Autodesk Inventor part; units mm, degrees
ref_plane "Work Plane2" through (31.1532, -17.5901, -37) normal (0.7071, 0.7071, 0) x (-0.7071, 0.7071, 0)
ref_plane "Work Plane4" through (0.92, 19.6401, -37) normal (-1, 0, 0) x (0, 0, -1)
ref_plane "YZ Plane" through (0, 0, 0) normal (1, 0, 0) x (0, 1, 0)
sketch "Sketch1" plane through (0, 0, 0) normal (0, 0, 1) x (1, 0, 0)
  line L0 (0, 0) -> (0, 7.4776)
  line L1 (0, 7.4776) -> (-5.7, 7.4776)
  line L2 (-5.7, 7.4776) -> (-21.2563, -8.0788)
  line L3 (-21.2563, -8.0788) -> (-21.2563, -11.0788)
  line L4 (-21.2563, -11.0788) -> (-20.5492, -11.7859)
  line L5 (-20.5492, -11.7859) -> (-21.2563, -12.493)
  line L6 (-21.2563, -12.493) -> (-19.7664, -13.983)
  line L7 (-19.7664, -13.983) -> (-25.1404, -19.357)
  line L8 (-25.1404, -19.357) -> (-27.1017, -19.2987)
  line L9 (-27.1017, -19.2987) -> (-27.8088, -20.0059)
  line L10 (-27.8088, -20.0059) -> (-23.0005, -24.8142)
  line L11 (-23.0005, -24.8142) -> (-3.2015, -5.0152)
  line L12 (-1.88, 9.6426) -> (-1.2574, 11.8658)
  line L13 (-1.2574, 11.8658) -> (-2.8574, 11.8658)
  line L14 (-2.8574, 11.8658) -> (-5.5444, 9.1788)
  line L15 (-23.5149, -7.7918) -> (-6.5444, 9.1788)
  line L16 (-6.5444, 9.1788) -> (-5.5444, 9.1788)
  line L17 (-23.5149, -7.7918) -> (-23.5149, -11.7918)
  line L18 (-29.3132, -17.5901) -> (-23.5149, -11.7918)
  line L19 (-29.3132, -17.5901) -> (-30.4446, -16.4587)
  line L20 (-30.4446, -16.4587) -> (-29.4153, -15.4295)
  line L21 (-29.4153, -15.4295) -> (-30.1224, -14.7223)
  line L22 (-30.1224, -14.7223) -> (-32.668, -17.2679)
  line L23 (-32.668, -17.2679) -> (-22.9298, -27.0062)
  line L24 (-22.9298, -27.0062) -> (-1.4337, -5.5102)
  line L25 (0.92, 16.812) -> (0.92, -19.9546) construction
  line L26 (1.84, 0) -> (1.84, 7.4776)
  line L27 (1.84, 7.4776) -> (7.54, 7.4776)
  line L28 (7.54, 7.4776) -> (23.0963, -8.0788)
  line L29 (23.0963, -8.0788) -> (23.0963, -11.0788)
  line L30 (23.0963, -11.0788) -> (22.3892, -11.7859)
  line L31 (22.3892, -11.7859) -> (23.0963, -12.493)
  line L32 (23.0963, -12.493) -> (21.6064, -13.983)
  line L33 (21.6064, -13.983) -> (26.9804, -19.357)
  line L34 (26.9804, -19.357) -> (28.9417, -19.2987)
  line L35 (28.9417, -19.2987) -> (29.6488, -20.0059)
  line L36 (29.6488, -20.0059) -> (24.8405, -24.8142)
  line L37 (24.8405, -24.8142) -> (5.0415, -5.0152)
  line L38 (3.72, 9.6426) -> (3.0974, 11.8658)
  line L39 (3.0974, 11.8658) -> (4.6974, 11.8658)
  line L40 (4.6974, 11.8658) -> (7.3844, 9.1788)
  line L41 (25.3549, -7.7918) -> (8.3844, 9.1788)
  line L42 (8.3844, 9.1788) -> (7.3844, 9.1788)
  line L43 (25.3549, -7.7918) -> (25.3549, -11.7918)
  line L44 (31.1532, -17.5901) -> (25.3549, -11.7918)
  line L45 (31.1532, -17.5901) -> (32.2846, -16.4587)
  line L46 (32.2846, -16.4587) -> (31.2553, -15.4295)
  line L47 (31.2553, -15.4295) -> (31.9624, -14.7223)
  line L48 (31.9624, -14.7223) -> (34.508, -17.2679)
  line L49 (34.508, -17.2679) -> (24.7698, -27.0062)
  line L50 (24.7698, -27.0062) -> (3.2737, -5.5102)
  line L51 (-1.88, 9.6426) -> (3.72, 9.6426)
  arc A0 (3.2737, -5.5102) -> (-1.4337, -5.5102) centre (0.92, -4.1167) ccw
  arc A1 (5.0415, -5.0152) -> (1.84, 0) centre (0.92, -4.1167) ccw
  arc A2 (0, 0) -> (-3.2015, -5.0152) centre (0.92, -4.1167) ccw
  point P0 (-22.4534, -16.67)
  dimension "d1" = 5.7
  dimension "d2" = 135
  dimension "d3" = 22
  dimension "d13" = 3
  dimension "d14" = 28
  dimension "d22" = 1.6
  dimension "d23" = 3.8
  dimension "d24" = 1
  dimension "d25" = 24
  dimension "d30" = 4
  dimension "d34" = 3.6
  dimension "d36" = 1.5
  dimension "d38" = 1.6
  dimension "d47" = 1.84
  dimension "d55" = 8.2
  dimension "d56" = 1.6
  dimension "d57" = 1
  dimension "d59" = 7.6
  dimension "d61" = 1
  dimension "d62" = 6.8
  dimension "d72" = 30.4
  dimension "d74" = 13.772
  dimension "d75" = 4.2
  dimension "d76" = 5.6
  dimension "d77" = 1.8
  dimension "d78" = 1
  dimension "d80" = 90
  dimension "d89" = 7.4776
extrude "Extrusion1" add sketch "Sketch1" against normal blind 37
ref_plane "Work Plane2" through (31.1532, -17.5901, -37) normal (0.7071, 0.7071, 0) x (-0.7071, 0.7071, 0)
sketch "Sketch3" plane through (31.1532, -17.5901, -37) normal (0.7071, 0.7071, 0) x (-0.7071, 0.7071, 0)
  circle A0 centre (5.2, 18.5) radius 3
  line L0 (0, 37) -> (8.2, 37)
  line L1 (8.2, 37) -> (8.2, 0)
  point P0 (34.4667, 37)
  dimension "d65" = 18.5
  dimension "d67" = 6
extrude "Extrusion2" cut sketch "Sketch3" against normal blind 6
thread "Thread1"
ref_plane "Work Plane4" through (0.92, 19.6401, -37) normal (-1, 0, 0) x (0, 0, -1)
mirror "Mirror2" about plane through (0.92, 19.6401, -37) normal (-1, 0, 0) of "Extrusion2"
thread "Thread2"
sketch "Sketch4" plane through (31.1532, -17.5901, -37) normal (0.7071, 0.7071, 0) x (-0.7071, 0.7071, 0)
  line L0 (4.95, 0) -> (4.95, 37)
  line L1 (27.3556, 0) -> (-0.6444, 0)
  line L2 (0, 37) -> (8.2, 37)
  line L3 (5.45, 0) -> (5.45, 37)
  line L4 (8.2, 37) -> (8.2, 18.5)
  line L5 (5.45, 37) -> (4.95, 37)
  line L6 (5.45, 0) -> (4.95, 0)
  point P0 (34.4667, 37)
  point P1 (4.95, 0)
  dimension "d84" = 2.75
  dimension "d85" = 0.5
extrude "Extrusion3" cut sketch "Sketch4" against normal blind 0.5
mirror "Mirror3" about plane through (0.92, 19.6401, -37) normal (-1, 0, 0) of "Extrusion3"
properties part number "ESCUADRA" material "Aluminum"
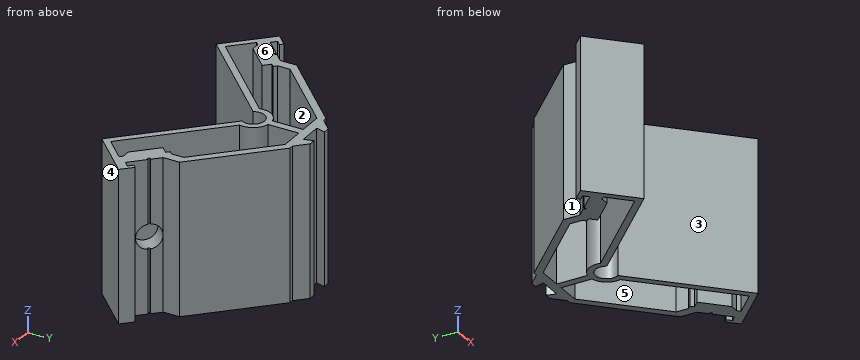
Could you check a few things on this model? Use its own coordinates, in mm. Face numbers are marked on the shaded views. A direction names the side the tool comes from. Round coordinates to 2 decimals unless told otherwise and drop trailing zeros. Loops run counter-clockwise (first coordinate to the right, second up) from the corner with the lowest first, then second, coordinate; pieces in that order, holes last. Notation, with made-up numbers: M -38.75,13.25 L -34.75,13.25 A15 cw -34.75,22.25 Z; hole C 8.25,15 d7. An arc over 180 degrees is marked long. Answer as CSV lines item,"result".
1) For pin 1 Ø8 at (y, z) = (-10, -6) entering from -X; pin 2 Ø6.5 at (x, z) = (-3.5, -12) entering from -Y; pin 3 Ø2 at (y, z) = (4.5, -13.5) entering from -X, each with a flat end and sliding along its axis, tell me the tip position at first contact or that it passes through.
From the geometry:
pin 1,"x = -25.46"
pin 2,"y = -10.83"
pin 3,"x = -12.22"
2) Imagine slicing it at D-D on z = -3.5. Count the separate pieces of the cut face and the enclosed holes in it, and give its area (3 significant figures).
From the geometry:
separate pieces,"1"
enclosed holes,"2"
area,"391 mm^2"
3) We'd pull the mould along X, two halves only. Please class the marked faces 4, 5 and 6: released by +X, released by -X, zero draft, split by the parting line, or undercut.
From the geometry:
face 4,"released by +X"
face 5,"undercut"
face 6,"zero draft"
4) Imagine slicing it at A-A on y = -3. List the corners of the cut face in (x, z) for me, and give its area (3 significant figures).
From the geometry:
outline,"M -18.72,-37 L -16.18,-37 L -16.18,0 L -18.72,0 Z; M -3.15,-37 L -1.58,-37 L -1.58,0 L -3.15,0 Z; M 3.42,-37 L 4.99,-37 L 4.99,0 L 3.42,0 Z; M 18.02,-37 L 20.56,-37 L 20.56,0 L 18.02,0 Z"
area,"305 mm^2"
5) Imagine slicing it at B-B on x = -9.5. List the corners of the cut face in (y, z) for me, and give its area (3 significant figures).
From the geometry:
outline,"M -13.58,-37 L -11.31,-37 L -11.31,0 L -13.58,0 Z; M 3.68,-37 L 6.22,-37 L 6.22,0 L 3.68,0 Z"
area,"178 mm^2"
6) Which directions (+Z, -Z, +X, -X, +Y, -Y) give clear straight access to the entire face, cutting with the end or side of a thin tool? Please do the marked faces 1, 2 and 3.
From the geometry:
face 1,"+Z, -Z, -X, +Y"
face 2,"+Z, -Z"
face 3,"+Z, -Z, -Y"
7) Imagine slicing it at C-C on y = 4. List the corners of the cut face in (x, z) for me.
From the geometry:
outline,"M -11.72,-37 L -9.18,-37 L -9.18,0 L -11.72,0 Z; M 0,-37 L 1.84,-37 L 1.84,0 L 0,0 Z; M 11.02,-37 L 13.56,-37 L 13.56,0 L 11.02,0 Z"
8) If I drill on probe 1 along X at (y, z) = (-17, -17); probe 2 along X at (y, z) = (-23.5, -8); probe 3 along X at (y, z) = (-9, -16.5), over which ranges is the centre line in solid material (lowest first)?
From the geometry:
probe 1,"-32.4 to -29.9, -28.72 to -26.22, -15.19 to -12.92, 14.76 to 17.03, 28.06 to 30.56, 31.74 to 34.24"
probe 2,"-26.44 to -24.31, -21.69 to -19.42, 21.26 to 23.53, 26.15 to 28.28"
probe 3,"-23.51 to -21.26, -7.19 to -4.92, 6.76 to 9.03, 23.1 to 25.35"
